For this review, take the finished solid that the model builds, in its own axes (mm). Give positions to 0.01 mm unless a question says otherwise; leave off trailing zeros. Write each loop counter-clockwise with the first axis right and the second up, starting at its lowest first coordinate (ties: lowest second). Pieces come first, ordered by that corner, then holes.
from build123d import *

# Parameters (mm, degrees)
SKETCH1_W           = 16
SKETCH1_H           = 20.5
SKETCH1_R           = 1.5
BOSS_EXTRUDE1_DEPTH = 1
SKETCH2_R           = 0.75
CUT_EXTRUDE2_DEPTH  = 14.040801356


with BuildPart() as part:
    # Sketch1 → Boss-Extrude1 (new body)
    with BuildSketch(Plane(origin=(0, 0, 0), x_dir=(1, 0, 0), z_dir=(0, 1, 0))):
        Rectangle(SKETCH1_W, SKETCH1_H)
        with Locations(Location((5.5, 7.5, 0), (0, 0, 270))):
            Circle(SKETCH1_R, mode=Mode.SUBTRACT)
        with Locations(Location((5.5, -7.5, 0), (0, 0, 270))):
            Circle(SKETCH1_R, mode=Mode.SUBTRACT)
    extrude(amount=BOSS_EXTRUDE1_DEPTH)

    # Sketch2 → Cut-Extrude2 (cut, through all)
    with BuildSketch(Plane(origin=(0, 1, 0), x_dir=(1, 0, 0), z_dir=(0, 1, 0))):
        with Locations(Location((-6, 8.75, 0), (0, 0, 270))):
            Circle(SKETCH2_R)
        with Locations(Location((-6, 6.25, 0), (0, 0, 270))):
            Circle(SKETCH2_R)
        with Locations(Location((-6, 3.75, 0), (0, 0, 270))):
            Circle(SKETCH2_R)
        with Locations(Location((-6, 1.25, 0), (0, 0, 270))):
            Circle(SKETCH2_R)
        with Locations(Location((-6, -1.25, 0), (0, 0, 270))):
            Circle(SKETCH2_R)
        with Locations(Location((-6, -3.75, 0), (0, 0, 270))):
            Circle(SKETCH2_R)
        with Locations(Location((-6, -6.25, 0), (0, 0, 270))):
            Circle(SKETCH2_R)
        with Locations(Location((-6, -8.75, 0), (0, 0, 270))):
            Circle(SKETCH2_R)
    extrude(amount=-CUT_EXTRUDE2_DEPTH, mode=Mode.SUBTRACT)


solid = part.part
(1) We need section A-A (z = 7.5). Write out the cut boundary in (x, y).
(2) We need section C-C (y = 0.55). Count the separate pieces of the cut face and the enclosed holes in it, and give its area (3 significant figures).
(3) We need section B-B (x = 5.5). Write out the cut boundary in (y, z).
(4) We need section D-D (z = 3.75). Write out the cut boundary in (x, y).
(5) For L1, parallel to X at y = 0.3, z = -1.25; L2, parallel to X at y = 0.7, z = -8.75; L3, parallel to X at y = 0.6, z = 7.5, list the stretches that pass through material, from the lowest coordinate up.
(6) The part is to be moulded in two halves that separate along X. For faces 1 (the cylindrical face through (-6, 0.5, 3)), 2 (the flat face through (-8, 0.5, 0.1)), 3 (the flat face through (8, 0.5, 0.1)), 4 (the flat face through (0, 0, 0)), say which applies: +X half, -X half, draft (parallel to the pull), parting line (faces both ways), or undercut.
The answers:
1. outline: (-8, 0) - (4, 0) - (4, 1) - (-8, 1) - close; (7, 0) - (8, 0) - (8, 1) - (7, 1) - close
2. separate pieces: 1
2. enclosed holes: 10
2. area: 300 mm2
3. outline: (0, -10.25) - (1, -10.25) - (1, -9) - (0, -9) - close; (0, -6) - (1, -6) - (1, 6) - (0, 6) - close; (0, 9) - (1, 9) - (1, 10.25) - (0, 10.25) - close
4. outline: (-8, 0) - (-6.75, 0) - (-6.75, 1) - (-8, 1) - close; (-5.25, 0) - (8, 0) - (8, 1) - (-5.25, 1) - close
5. L1: x = -8 to -6.75, -5.25 to 8
5. L2: x = -8 to -6.75, -5.25 to 4.67, 6.33 to 8
5. L3: x = -8 to 4, 7 to 8
6. face 1: undercut
6. face 2: -X half
6. face 3: +X half
6. face 4: draft
